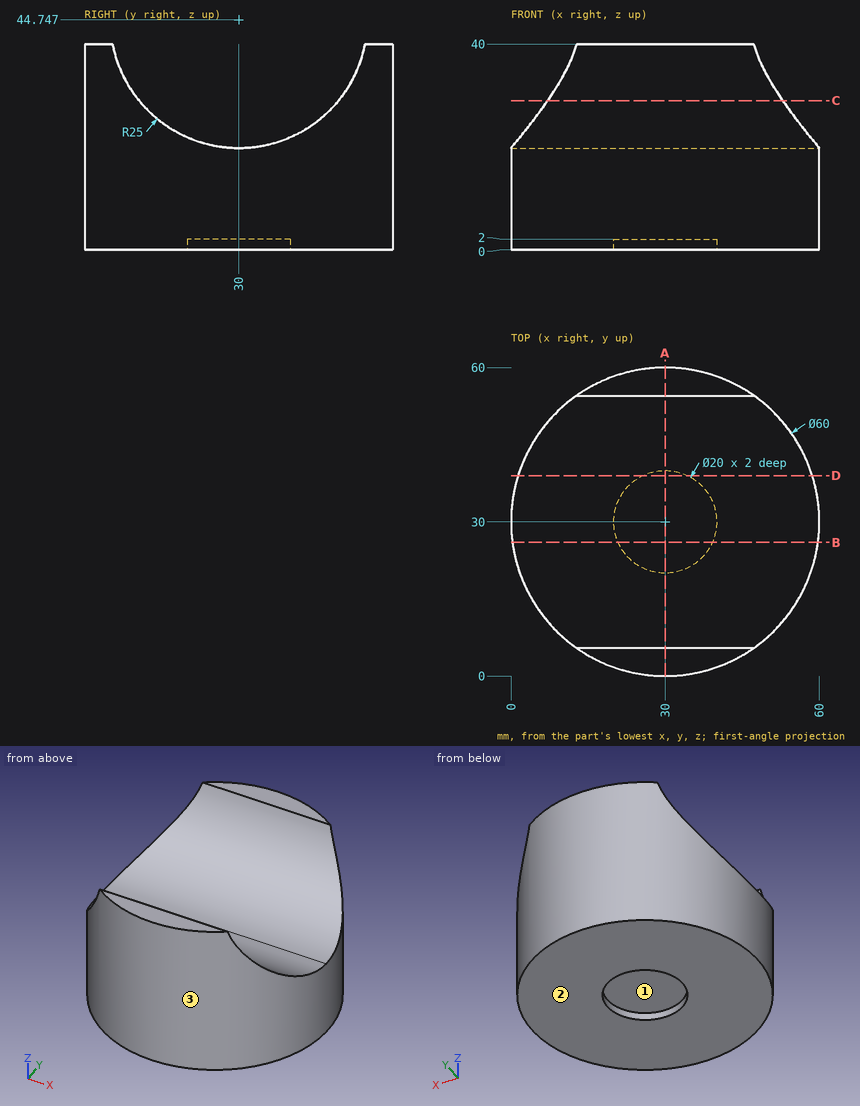
For this review, use the dimensioned drawing (mm, ordinates from the lowest corner) and the shaded views. Give positions to 0.01 mm unless a question says otherwise; leave off trailing zeros. Write each loop counter-clockwise with the first axis right and the second up, starting at its lowest first coordinate (ties: lowest second). Pieces come first, ordered by that corner, then holes. Notation, with made-up numbers: M 33,81 L 68,81 A19 cw 68,95 Z; hole C 31.5,-30.75 d11. An arc over 180 degrees is marked long. Answer as a JSON object with one key per item and string values. Group by question number.
1) For line 1 along Y through (x, z) = (30, 1.2); line 2 along Y through (x, z) = (31.5, 32); line 3 along X through (y, z) = (29, 12), list the stretches that pass through material, from the lowest coordinate up.
2) We need section C-C (z = 29). Give the boundary of the cut face in (x, y).
3) We need section D-D (y = 39). Give the boundary of the cut face in (x, z).
4) We need section B-B (y = 26). Give the boundary of the cut face in (x, z) (3 decimals).
5) Mouldability with a two-part tool opening along Y and no side actions: class the marked faces 1, 2 and 3 as released by +Y, released by -Y, zero draft, split by the parting line, or undercut.
6) We need section A-A (x = 30). Give the boundary of the cut face in (y, z) (1 decimal).
7) Clearance check with flat-ended pins moving along their axes: pin 1 Ø1 at (x, z) = (21, 22) entering from -Y; pin 2 Ø8 at (y, z) = (7.5, 4) entering from -X; pin 3 Ø16 at (x, y) = (30, 30) entering from -Z; pin 4 Ø16 at (x, y) = (34, 33) entering from -Z. State where each tip first meets the part, or that it passes through.
Answer key:
{
 "1": {"line 1": "y = 0 to 20, 40 to 60", "line 2": "y = 0.04 to 8.49, 51.51 to 59.96", "line 3": "x = 0.02 to 59.98"},
 "2": {"outline": "M 7.13,10.58 A30 ccw 52.87,10.58 Z; M 7.13,49.42 L 52.87,49.42 A30 ccw Z"},
 "3": {"outline": "M 1.38,0 L 25.64,0 L 25.64,2 L 34.36,2 L 34.36,0 L 58.62,0 L 58.62,21.42 L 1.38,21.42 Z"},
 "4": {"outline": "M 0.268,0 L 20.835,0 L 20.835,2 L 39.165,2 L 39.165,0 L 59.732,0 L 59.732,20.069 L 0.268,20.069 Z"},
 "5": {"face 1": "undercut", "face 2": "zero draft", "face 3": "split by the parting line"},
 "6": {"outline": "M 0,0 L 20,0 L 20,2 L 40,2 L 40,0 L 60,0 L 60,40 L 54.5,40 A25 cw 5.5,40 L 0,40 Z"},
 "7": {"pin 1": "stops at y = 1.23", "pin 2": "stops at x = 6.38", "pin 3": "stops at z = 2", "pin 4": "stops at z = 0"}
}
